The model under review builds one solid part; all positions refer to its coordinate system, in mm. Face numbers are marked on the shaded views. A direction names the side the tool comes from. Round coordinates to 2 decimals unless told otherwise and drop trailing zeros. Order: outer loops, then holes, each group sorted by start corner. A loop starts at its lowest first (then second) coordinate and runs counter-clockwise, first axis right, second up. Notation, with made-up numbers: M 89,75 L 110,75 A13 ccw 110,79 Z; hole C 88,29.25 d4. An arc over 180 degrees is marked long. Answer as a JSON object with one key per item and string values. Group by question number.
1. Clearance check with flat-ended pins moving along their axes: P1, Ø12.5, axis at y = 52, z = 47, coming from the -X side; P2, Ø4, axis at x = 1.5, z = 21.5, coming from the +Y side; P3, Ø4.5, axis at x = 19, y = 13.5, coming from the +Z side. State where each tip first meets the part, or that it passes through.
2. Mouldability with a two-part tool opening along X and no side actions: class the marked faces 1, 2 and 3 as released by +X, released by -X, zero draft, split by the parting line, or undercut.
3. Add section C-C on z = 18.5. State the section outline as (x, y) points, and give its area (3 significant figures).
4. Machinability: for the marked faces 4, 5, 6, 7 and 8, which of the approach directions +Z, -Z, +X, -X, +Y, -Y give a long, thin tool a straight path to every point of the face, cutting with its end or side? Answer none if there is none.
5. To check wall thickness, follow probe 1 along Y at (x, z) = (-33, 36); probe 2 along Z at (x, y) = (-13.5, 16.5); probe 3 along Y at (x, z) = (-37, 55). State the ranges of each line that lie inside material, in increasing order. Write a range as [from, to].
6. Add section B-B on y = 41. State the section outline as (x, z) points, and give its area (3 significant figures).
7. Add section A-A on x = 18.5. State the section outline as (y, z) points, and give its area (3 significant figures).
8. Add section D-D on y = 0. State the section outline as (x, z) points.
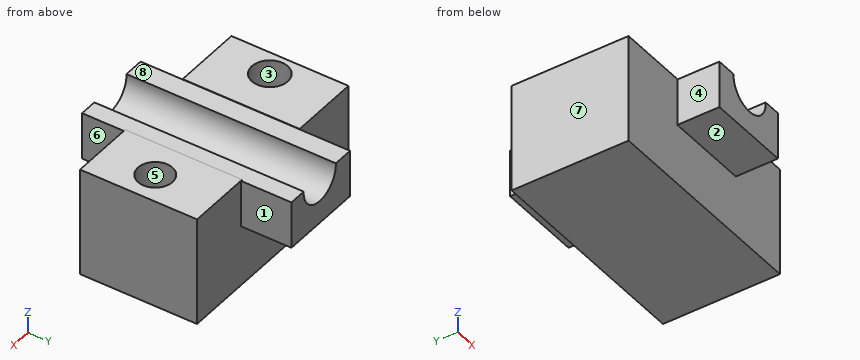
```python
from build123d import *

# Parameters (mm, degrees)
F0_W     = 116.026688
F0_H     = 62.326629
F1_DEPTH = 57.912
F2_R     = 9.178943
F2_R_2   = 9.568462
F3_DEPTH = 25.4
F4_W     = 44.070687
F4_H     = 119.394876
F5_DEPTH = 25.4
F6_W     = 44.824161
F6_H     = 111.522015
F7_DEPTH = 25.146
F9_DEPTH = 139.446


with BuildPart() as f1:
    # F0 (on Top) → F1 (new body)
    with BuildSketch(Plane.XY):
        with Locations((1.10502, 2.008145)):
            Rectangle(F0_W, F0_H)
    extrude(amount=F1_DEPTH)

    # F2 (on face) → F3 (cut)
    with BuildSketch(Plane.XY.offset(57.912)):
        with Locations((43.431606, 0)):
            Circle(F2_R)
        with Locations((-44.370782, 0)):
            Circle(F2_R_2)
    extrude(amount=-F3_DEPTH, mode=Mode.SUBTRACT)

    # F4 (on face) → F5 (cut)
    with BuildSketch(Plane.XY.offset(57.912)):
        with Locations((2.529694, -0.217967)):
            Rectangle(F4_W, F4_H)
    extrude(amount=-F5_DEPTH, mode=Mode.SUBTRACT)

    # F6 (on face) → F7 (join)
    with BuildSketch(Plane.XY.offset(32.512)):
        with Locations((2.90643, 4.208925)):
            Rectangle(F6_W, F6_H)
    extrude(amount=F7_DEPTH)

    # F8 (on face) → F9 (cut)
    with BuildSketch(Plane.XZ.offset(51.552083)):
        with BuildLine():
            Line((15.938878, 57.658), (-8.679586, 57.658))
            ThreePointArc((-8.679586, 57.658), (3.629646, 44.618661), (15.938878, 57.658))
        make_face()
    extrude(amount=-F9_DEPTH, mode=Mode.SUBTRACT)


solid = f1.part
```
Recorded:
{
 "1": {"P1": "stops at x = -19.51", "P2": "stops at y = 33.17", "P3": "stops at z = 57.66"},
 "2": {"face 1": "released by +X", "face 2": "zero draft", "face 3": "undercut"},
 "3": {"outline": "M -56.91,-29.16 L 59.12,-29.16 L 59.12,33.17 L -56.91,33.17 Z", "area": "7,230 mm²"},
 "4": {"face 4": "+Z, -Z, -X, -Y", "face 5": "+Z", "face 6": "+Z, -Z, +X, -Y", "face 7": "+Z, -Z, -X, +Y, -Y", "face 8": "+Z, +Y, -Y"},
 "5": {"probe 1": "y = [-29.16, 33.17]", "probe 2": "z = [0, 57.66]", "probe 3": "y = [-29.16, -6.1], [6.1, 33.17]"},
 "6": {"outline": "M -19.51,32.51 L 25.32,32.51 L 25.32,57.66 L 15.94,57.66 A12.33 cw long -8.68,57.66 L -19.51,57.66 Z", "area": "871 mm²"},
 "7": {"outline": "M -51.55,32.51 L -29.16,32.51 L -29.16,0 L 33.17,0 L 33.17,32.51 L 59.97,32.51 L 59.97,57.66 L -51.55,57.66 Z", "area": "4,830 mm²"},
 "8": {"outline": "M -56.91,0 L 59.12,0 L 59.12,57.91 L 52.61,57.91 L 52.61,32.51 L 34.25,32.51 L 34.25,57.91 L 24.57,57.91 L 24.57,57.66 L 15.94,57.66 A12.33 cw long -8.68,57.66 L -19.51,57.66 L -19.51,57.91 L -34.8,57.91 L -34.8,32.51 L -53.94,32.51 L -53.94,57.91 L -56.91,57.91 Z"}
}
